Input: part model. Units: mm. Frame: model coordinates. A direction names the side the tool comes from. Coordinates: 2 decimals unless noted, no trailing zeros. Loops run counter-clockwise (first coordinate to the right, second up) from the corner with the lowest first, then second, coordinate; pieces in that order, holes last. Notation, with made-up numbers: (-3, 36) - (45, 36) arc R15 ccw to (45, 54) - close; hole circle Ø6 at (75, 36.25). An arc over 180 degrees is marked (long way). Use one line per item in the form item = value.
from build123d import *

# Parameters (mm, degrees)
BOSS_EXTRUDE1_DEPTH  = 8
SKETCH2_R            = 4
CUT_EXTRUDE1_DEPTH   = 45
CUT_EXTRUDE1_TAPER   = 5
SKETCH3_R            = 2.1
BOSS_EXTRUDE2_DEPTH  = 3
FILLET1_R            = 2
FILLET1_OF_MIRROR1_R = 2


with BuildPart() as part:
    # Sketch1 → Boss-Extrude1 (new body, symmetric)
    with BuildSketch(Plane.XY):
        Polygon((-60.9, 0), (-60.9, 107), (0, 151.8745296), (60.9, 107), (60.9, 0), (44.9, 0), (44.9, 98.91516619), (0, 132), (-44.9, 98.91516619), (-44.9, 0), align=None)
    extrude(amount=BOSS_EXTRUDE1_DEPTH, both=True)

    # Sketch2 → Cut-Extrude1 (cut)
    with BuildSketch(Plane.XZ):
        with Locations((-60.9, 8)):
            Circle(SKETCH2_R)
        with Locations((-44.9, 8)):
            Circle(SKETCH2_R)
    cut_extrude1 = extrude(amount=-CUT_EXTRUDE1_DEPTH, taper=CUT_EXTRUDE1_TAPER, mode=Mode.SUBTRACT)

    # Sketch3 → Boss-Extrude2 (add)
    with BuildSketch(Plane.XZ):
        Polygon((-60.9, -8), (-68.936989859, 4.1), (-68.936989859, 16.1), (-36.863010141, 16.1), (-36.863010141, 4.1), (-44.9, -8), align=None)
        with Locations((-60.836989859, 8)):
            Circle(SKETCH3_R, mode=Mode.SUBTRACT)
        with Locations((-44.9, 8)):
            Circle(SKETCH3_R, mode=Mode.SUBTRACT)
    boss_extrude2 = extrude(amount=BOSS_EXTRUDE2_DEPTH)

    # Fillet1
    fillet1_edges = [part.edges().sort_by_distance(p)[0] for p in [
        (-36.863010141, -1.5, 4.1),
        (-36.863010141, -1.5, 16.1),
        (-68.936989859, -1.5, 16.1),
        (-68.936989859, -1.5, 4.1),
    ]]
    fillet(fillet1_edges, radius=FILLET1_R)

    # Mirror1: Cut-Extrude1, Boss-Extrude2 across plane
    add(cut_extrude1.mirror(Plane(origin=(0, 0, 0), x_dir=(0, 0, 1), z_dir=(1, 0, 0))), mode=Mode.SUBTRACT)
    add(boss_extrude2.mirror(Plane(origin=(0, 0, 0), x_dir=(0, 0, 1), z_dir=(1, 0, 0))))

    # Fillet1 of Mirror1
    fillet1_of_mirror1_edges = [part.edges().sort_by_distance(p)[0] for p in [
        (36.863010141, -1.5, 4.1),
        (36.863010141, -1.5, 16.1),
        (68.936989859, -1.5, 16.1),
        (68.936989859, -1.5, 4.1),
    ]]
    fillet(fillet1_of_mirror1_edges, radius=FILLET1_OF_MIRROR1_R)


solid = part.part
Q1. First-contact query: P1, Ø8, axis at y = 44, z = 0, coming from the +X side; P2, Ø12, axis at x = 51.5, z = -1, coming from the +Y side; P3, Ø12, axis at x = -55.5, z = 1, coming from the +Y side; P4, Ø5, axis at x = 60.84, z = 8, coming from the -Y side. Flat tips, straight axial feed; report the tip coordinate or a pass-through.
Check values:
P1 = 60.9
P2 = 118.35
P3 = 115.4
P4 = -3
Q2. Pull-direction query (Y, two-part tool) for faces 1 (the flat face through (-53, 0, 10)), 2 (the cylindrical face through (46.448, -1.479, 9.419)), 3 (the flat face through (53, -3, 4)); classes: pulls with the +Y half, pulls with the -Y half, needs draft (parallel to the pull), parting line crosses it, or undercut.
Check values:
face_1 = undercut
face_2 = needs draft
face_3 = pulls with the -Y half
Q3. Cut plane C-C, the plane z = 1.5. Return loops of the section in (x, y).
Check values:
outline = (-67.21, -3) - (-38.59, -3) - (-38.59, 0) - (-44.9, 0) - (-44.9, 98.92) - (0, 132) - (44.9, 98.92) - (44.9, 0) - (38.59, 0) - (38.59, -3) - (67.21, -3) - (67.21, 0) - (60.9, 0) - (60.9, 107) - (0, 151.87) - (-60.9, 107) - (-60.9, 0) - (-67.21, 0) - close
Q4. Set-up query: faces 4 (the cylindrical face through (62.4, -1.5, 9.4)), 5 (the flat face through (60.9, 54, 0)), 6 (the flat face through (40.995, -1.479, -2.12)), 7 (the conical face through (-46.332, 22.815, 6.599)), 8 (the flat face through (44.9, 49, 0)). Return all of +Z, -Z, +X, -X, +Y, -Y with unobstructed straight access to the full face (end or side cutting, diameter ignored); none if empty.
Check values:
face_4 = -Y
face_5 = +Z, -Z, +X, +Y
face_6 = -Z, -Y
face_7 = +Z
face_8 = +Z, -Z
Q5. Cut plane B-B, the plane z = 12. Return loops of the section in (x, y), then the cut area to 3 significant figures.
Check values:
outline = (-68.94, -3) - (-36.86, -3) - (-36.86, 0) - (-68.94, 0) - close; (36.86, -3) - (68.94, -3) - (68.94, 0) - (36.86, 0) - close
area = 192 mm²
Q6. Cut plane A-A, the plane y = 61.5. Return loops of the section in (x, z), then the cut area to 3 significant figures.
Check values:
outline = (-60.9, -8) - (-44.9, -8) - (-44.9, 8) - (-60.9, 8) - close; (44.9, -8) - (60.9, -8) - (60.9, 8) - (44.9, 8) - close
area = 512 mm²
Q7. Ray query, line 1 along X through (y, z) = (64.5, 4); line 2 along Z through (x, y) = (-33, 118.5); line 3 along Y through (x, z) = (-38.5, 3.75). Return the intervals inside material, ascending. Write a range as [from, to].
Check values:
line_1 = [-60.9, -44.9], [44.9, 60.9]
line_2 = [-8, 8]
line_3 = [-3, 0], [103.63, 123.51]
Q8. Cut plane D-D, the plane y = 8.5. Return loops of the section in (x, z), then the cut area to 3 significant figures.
Check values:
outline = (-60.9, -8) - (-44.9, -8) - (-44.9, 4.74) arc R3.26 cw to (-48.16, 8) - (-57.64, 8) arc R3.26 cw to (-60.9, 4.74) - close; (44.9, -8) - (60.9, -8) - (60.9, 4.74) arc R3.26 cw to (57.64, 8) - (48.16, 8) arc R3.26 cw to (44.9, 4.74) - close
area = 479 mm²
